```python
from build123d import *

# Parameters (mm, degrees)
SKETCH1_W                              = 152.4
SKETCH1_H                              = 84.6074
EXTRUDE1_DEPTH                         = 55.88
TAPPED_HOLE_FOR_1_4_20_HELICOIL1_D     = 6.7564
TAPPED_HOLE_FOR_1_4_20_HELICOIL1_DEPTH = 19.685
TAPPED_HOLE_FOR_1_4_20_HELICOIL1_TIP   = 2.029827343
F_1_4_0_25_DIAMETER_HOLE1_D            = 6.35
F_1_4_0_25_DIAMETER_HOLE1_DEPTH        = 27.94
F_1_4_0_25_DIAMETER_HOLE1_TIP          = 1.907732465
CHAMFER1_SIZE                          = 5.08


with BuildPart() as part:
    # Sketch1 → Extrude1 (new body)
    with BuildSketch(Plane(origin=(0, 0, 0), x_dir=(1, 0, 0), z_dir=(0, 1, 0))):
        Rectangle(SKETCH1_W, SKETCH1_H)
    extrude(amount=EXTRUDE1_DEPTH)

    # Tapped Hole for 1/4-20 Helicoil1
    with Locations(Plane.XY.offset(42.3037)):
        with Locations((-38.1, 27.94), (38.1, 27.94)):
            Hole(TAPPED_HOLE_FOR_1_4_20_HELICOIL1_D / 2, depth=TAPPED_HOLE_FOR_1_4_20_HELICOIL1_DEPTH)
            with Locations((0, 0, -(TAPPED_HOLE_FOR_1_4_20_HELICOIL1_DEPTH + TAPPED_HOLE_FOR_1_4_20_HELICOIL1_TIP / 2))):  # 118° drill point
                Cone(0, TAPPED_HOLE_FOR_1_4_20_HELICOIL1_D / 2, TAPPED_HOLE_FOR_1_4_20_HELICOIL1_TIP, mode=Mode.SUBTRACT)

    # 1/4 (0.25) Diameter Hole1
    with Locations(Plane(origin=(0, 55.88, 0), x_dir=(-1, 0, 0), z_dir=(0, 1, 0))):
        with Locations((-38.160987939, 25.011375754), (38.039012061, 25.011375754)):
            Hole(F_1_4_0_25_DIAMETER_HOLE1_D / 2, depth=F_1_4_0_25_DIAMETER_HOLE1_DEPTH)
            with Locations((0, 0, -(F_1_4_0_25_DIAMETER_HOLE1_DEPTH + F_1_4_0_25_DIAMETER_HOLE1_TIP / 2))):  # 118° drill point
                Cone(0, F_1_4_0_25_DIAMETER_HOLE1_D / 2, F_1_4_0_25_DIAMETER_HOLE1_TIP, mode=Mode.SUBTRACT)

    # Chamfer1
    chamfer1_edges = [part.edges().sort_by_distance(p)[0] for p in [
        (76.2, 55.88, 0),
        (-76.2, 55.88, 0),
        (76.2, 0, 0),
        (-76.2, 0, 0),
    ]]
    chamfer(chamfer1_edges, length=CHAMFER1_SIZE)


solid = part.part
```
The listing builds one solid part. Answer for the finished solid, in the listing's coordinates (mm). A direction names the side the tool comes from. Coordinates: 2 decimals unless noted, no trailing zeros. One line per item, written item: value.
1) A tool of negligible diameter and unlimited length cuts with its end or side. For faces 1 (the cylindrical face through (38.83, 24.64, 32.32)), 2 (the cylindrical face through (-36.574, 42.206, 22.195)), 3 (the flat face through (74, 53, 1)), from which of +Z, -Z, +X, -X, +Y, -Y can it reach the whole face along a straight path? Write none if from no direction.
Geometry check:
face 1: +Z
face 2: +Y
face 3: +Z, -Z, +X, +Y
2) For a pull along X with two mould halves and no side action, classify faces 4 (the conical face through (37.97, 27.37, 20.94)), 5 (the flat face through (-1, 28, 42.304)), 6 (the flat face through (73.7, 2.58, 0.59)), 7 (the cylindrical face through (39.626, 42.206, 22.195)) as pulls with the +X half, pulls with the -X half, needs draft (parallel to the pull), parting line crosses it, or undercut.
Geometry check:
face 4: undercut
face 5: needs draft
face 6: pulls with the +X half
face 7: undercut
3) Consider line 1 along X through (y, z) = (27.94, 37); line 2 along Y through (x, z) = (-38.1, 32.75); line 3 along X through (y, z) = (27, 31). Determine where each line is inside the solid, lowest interval first. Write a range as from..to.
Geometry check:
line 1: x = -76.2..-41.48, -34.72..34.72, 41.48..76.2
line 2: y = 0..24.56, 31.32..55.88
line 3: x = -76.2..-41.34, -34.86..34.86, 41.34..76.2
